Model file for the job. Use its own axes, mm. A direction names the side the tool comes from. Round coordinates to 2 decimals unless told otherwise and drop trailing zeros. Loops run counter-clockwise (first coordinate to the right, second up) from the corner with the lowest first, then second, coordinate; pieces in that order, holes last. Notation, with made-up numbers: M -0.75,-30 L 21.25,-30 A22 ccw 21.25,-9 Z; hole C 85,46 d9. An arc over 180 degrees is marked long. Use a Markdown table: item, result. Add a question column.
Item 1: Saw through at C-C on x = 20.5. Write the cut outline in (y, z).
Item 2: Pin check, flat tips, straight feed: P1, Ø1.2, axis at y = 6, z = -2, coming from the +X side; P2, Ø2, axis at x = 11.5, z = -2.5, coming from the +Y side; P3, Ø2.5, axis at x = 3, y = 6.5, coming from the -Z side; P4, Ø4.5, axis at x = 14.5, z = -3, coming from the -Y side. Stop position of each tip, or through.
Item 3: Saw through at D-D on z = -2.5. Write the cut outline in (x, y), then the cut area to 3 significant figures.
Item 4: Two-plate mould, pull along X, no slides. Class faces 5 (the flat face through (8.256, 5.759, 3.809)), 6 (the flat face through (23.073, 5.842, 3.91)), 7 (the flat face through (6.4, 6, -2)): +X half, -X half, draft (parallel to the pull), parting line (faces both ways), or undercut.
Item 5: Wall check: L1, parallel to X at y = 6.5, z = 0.55; L2, parallel to Y at x = 28, z = 0.45; L3, parallel to Z at x = 21, y = 9.25. Give the ranges that are in metal, low to high. Write a range as from..to.
Item 6: Saw through at A-A on x = 28. Write the cut outline in (y, z).
Item 7: Tool access for faces 1 (the cylindrical face through (22, 2, 4)), 2 (the flat face through (15, 0.8, -2)), 3 (the flat face through (15, 6, 0.9)), 4 (the flat face through (7.746, 5.752, 3.91)): list every direction of +Z, -Z, +X, -X, +Y, -Y with a clear straight run to the whole face (end or side of a thin tool).
Item 8: Saw through at B-B on z = 1.75. Write the cut outline in (x, y), then the cut area to 3 significant figures.
```python
from build123d import *

# Parameters (mm, degrees)
CYLINDER_R        = 1.5
CYLINDER_DEPTH    = 10
CYLINDER001_R     = 1.5
CYLINDER001_DEPTH = 10
BOX001_W          = 18
BOX001_H          = 11
BOX001_DEPTH      = 5.2
BOX_W             = 30.8
BOX_H             = 12.6
BOX_DEPTH         = 0.9
FILLET_R          = 1
FILLET001_R       = 1
PAD_DEPTH         = 5.9
FILLET002_R       = 0.2
FILLET003_R       = 1


with BuildPart() as cylinder:
    # Cylinder → Cylinder (new body)
    with BuildSketch(Plane.XY.offset(-2)):
        Circle(CYLINDER_R)
    extrude(amount=CYLINDER_DEPTH)


with BuildPart() as fusion:
    # Cylinder001 → Cylinder001 (new body)
    with BuildSketch(Plane(origin=(25, 0, -2), x_dir=(1, 0, 0), z_dir=(0, 0, 1))):
        Circle(CYLINDER001_R)
    extrude(amount=CYLINDER001_DEPTH)

    # Fusion: union Cylinder
    add(cylinder.part)


with BuildPart() as fusion_1:
    # Fusion placement: moved
    add(fusion.part.moved(Location((3, 6.5, 0))))


with BuildPart() as cube001:
    # Box001 → Box001 (new body)
    with BuildSketch(Plane(origin=(6.4, 0.8, -5), x_dir=(1, 0, 0), z_dir=(0, 0, 1))):
        with Locations((9, 5.5)):
            Rectangle(BOX001_W, BOX001_H)
    extrude(amount=BOX001_DEPTH)


with BuildPart() as fillet003:
    # Box → Box (new body)
    with BuildSketch(Plane.XY):
        with Locations((15.4, 6.3)):
            Rectangle(BOX_W, BOX_H)
    extrude(amount=BOX_DEPTH)

    # Fusion001: union Cube001
    add(cube001.part)

    # Cut: cut Fusion
    add(fusion_1.part, mode=Mode.SUBTRACT)

    # Fillet
    fillet_edges = [fillet003.edges().sort_by_distance(p)[0] for p in [
        (24.4, 0.8, -2.5),
        (24.4, 11.8, -2.5),
        (24.4, 6.3, -5),
        (6.4, 0.8, -2.5),
        (15.4, 0.8, -5),
        (6.4, 11.8, -2.5),
        (15.4, 11.8, -5),
        (6.4, 6.3, -5),
    ]]
    fillet(fillet_edges, radius=FILLET_R)

    # Fillet001
    fillet001_edges = [fillet003.edges().sort_by_distance(p)[0] for p in [
        (0, 0, 0.45),
        (0, 12.6, 0.45),
        (30.8, 12.6, 0.45),
        (30.8, 0, 0.45),
    ]]
    fillet(fillet001_edges, radius=FILLET001_R)

    # Sketch → Pad (new body)
    with BuildSketch(Plane.XY.offset(0.9)):
        Polygon((6.8, 10.204892), (24, 10.204892), (22.214525, 1.804892), (8.585475, 1.804892), align=None)
        Polygon((7.417449, 9.704892), (23.382551, 9.704892), (21.809633, 2.304892), (8.990367, 2.304892), align=None, mode=Mode.SUBTRACT)
    extrude(amount=PAD_DEPTH)

    # Fillet002
    fillet002_edges = [fillet003.edges().sort_by_distance(p)[0] for p in [
        (15.4, 10.204892, 0.9),
        (23.107262, 6.004892, 0.9),
        (15.4, 1.804892, 0.9),
        (7.692738, 6.004892, 0.9),
    ]]
    fillet(fillet002_edges, radius=FILLET002_R)

    # Fillet003
    fillet003_edges = [fillet003.edges().sort_by_distance(p)[0] for p in [
        (6.8, 10.204892, 3.95),
        (24, 10.204892, 3.95),
        (8.585475, 1.804892, 3.95),
        (22.214525, 1.804892, 3.95),
        (7.417449, 9.704892, 3.85),
        (23.382551, 9.704892, 3.85),
        (21.809633, 2.304892, 3.85),
        (8.990367, 2.304892, 3.85),
    ]]
    fillet(fillet003_edges, radius=FILLET003_R)


solid = fillet003.part
```
Entries:
| question | item | result |
|---|---|---|
| 1 | outline | M 0,0 L 0.8,0 L 0.8,-4 A1 ccw 1.8,-5 L 10.8,-5 A1 ccw 11.8,-4 L 11.8,0 L 12.6,0 L 12.6,0.9 L 10.4,0.9 A0.2 cw 10.2,1.1 L 10.2,6.8 L 9.7,6.8 L 9.7,0.9 L 2.3,0.9 L 2.3,6.8 L 1.8,6.8 L 1.8,1.1 A0.2 cw 1.6,0.9 L 0,0.9 Z |
| 2 | P1 | x = 24.4 |
| 2 | P2 | y = 11.8 |
| 2 | P3 | through |
| 2 | P4 | y = 0.8 |
| 3 | outline | M 6.4,1.8 A1 ccw 7.4,0.8 L 23.4,0.8 A1 ccw 24.4,1.8 L 24.4,10.8 A1 ccw 23.4,11.8 L 7.4,11.8 A1 ccw 6.4,10.8 Z |
| 3 | area | 197 mm2 |
| 4 | face 5 | undercut |
| 4 | face 6 | +X half |
| 4 | face 7 | -X half |
| 5 | L1 | 0..1.5, 4.5..26.5, 29.5..30.8 |
| 5 | L2 | 0..5, 8..12.6 |
| 5 | L3 | -5..0.9 |
| 6 | outline | M 0,0 L 5,0 L 5,0.9 L 0,0.9 Z; M 8,0 L 12.6,0 L 12.6,0.9 L 8,0.9 Z |
| 7 | face 1 | +Z, +X, -Y |
| 7 | face 2 | -Z, +X, -X, -Y |
| 7 | face 3 | +Z |
| 7 | face 4 | +Z, -X, -Y |
| 8 | outline | M 7.06,9 L 8.42,2.6 A1 ccw 9.4,1.8 L 21.4,1.8 A1 ccw 22.38,2.6 L 23.74,9 A1 ccw 22.77,10.2 L 8.03,10.2 A1 ccw Z; hole M 7.67,8.5 L 8.82,3.1 A1 ccw 9.8,2.3 L 21,2.3 A1 ccw 21.98,3.1 L 23.13,8.5 A1 ccw 22.15,9.7 L 8.65,9.7 A1 ccw Z |
| 8 | area | 23.0 mm2 |
